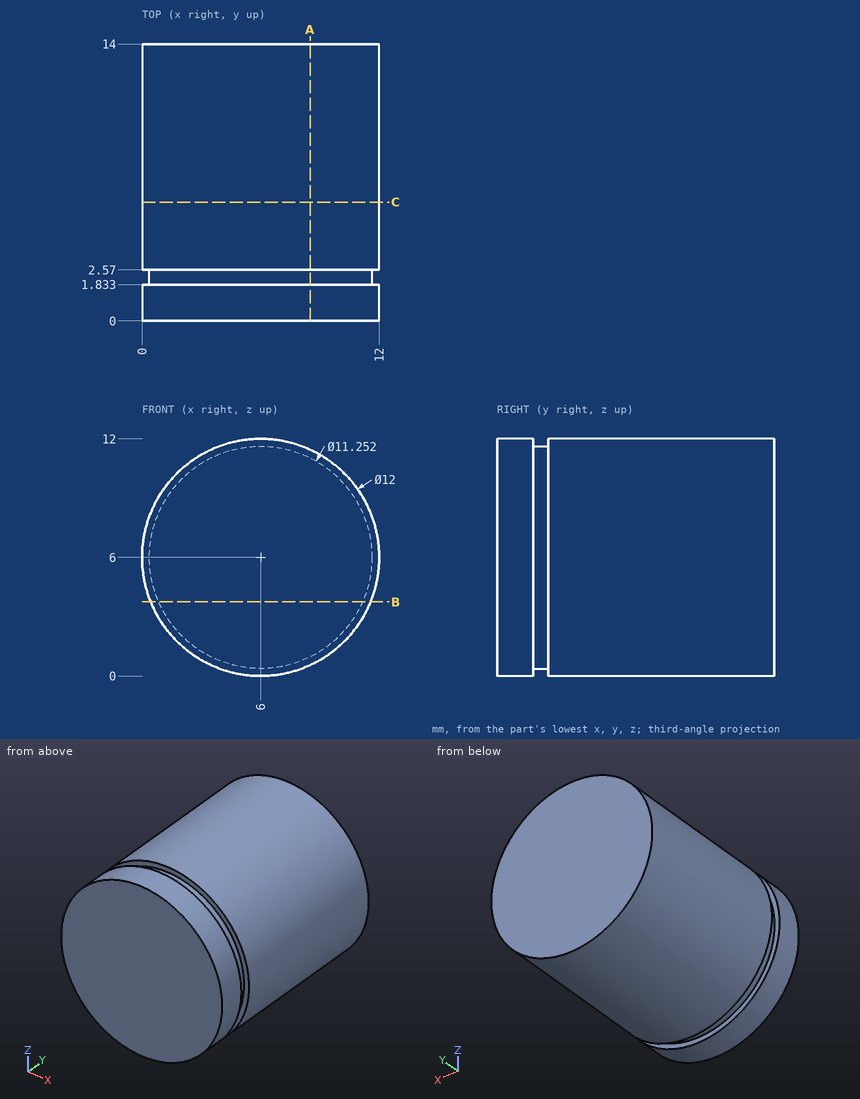
Answer from the drawing. Dimensions are ordinates in mm from the lowest x, y and z of the part. Round coordinates to 2 decimals unless told otherwise and drop trailing zeros. Loops run counter-clockwise (first coordinate to the right, second up) from the corner with the lowest first, then second, coordinate; pieces in that order, holes last.
Q1. Each of these flat-tipped pins is pushed along its axis until it touches: pin 1 (6 mm diameter, centred on y = 8, z = 2.5, fed in from +X); pin 2 (4 mm diameter, centred on y = 11, z = 3, fed in from -X); pin 3 (2 mm diameter, centred on y = 4, z = 10, fed in from +X). Where does it stop, or does it pass through?
Q2. Section C-C on y = 6 is taken. Write down the section's boundary in (x, z).
Q3. Section B-B on z = 3.75 is taken. Write down the section's boundary in (x, y).
Q4. Section A-A on x = 8.5 is taken. Write down the section's boundary in (y, z) (1 decimal).
Q5. Consider probe 1 along Z at (x, y) = (9.75, 2) (1 decimal); probe 2 along X at (y, z) = (11.5, 1) (1 decimal); probe 3 along X at (y, z) = (8, 2.25) (1 decimal). Determine where each line is inside the solid, lowest interval first.
Output:
1. pin 1: stops at x = 11.98
1. pin 2: stops at x = 0.08
1. pin 3: stops at x = 11.2
2. outline: circle Ø12 at (6, 6)
3. outline: (0.44, 0) - (11.56, 0) - (11.56, 1.83) - (11.16, 1.83) - (11.16, 2.57) - (11.56, 2.57) - (11.56, 14) - (0.44, 14) - (0.44, 2.57) - (0.84, 2.57) - (0.84, 1.83) - (0.44, 1.83) - close
4. outline: (0, 0.5) - (1.8, 0.5) - (1.8, 1) - (2.6, 1) - (2.6, 0.5) - (14, 0.5) - (14, 11.5) - (2.6, 11.5) - (2.6, 11) - (1.8, 11) - (1.8, 11.5) - (0, 11.5) - close
5. probe 1: z = 1.8 to 10.2
5. probe 2: x = 2.7 to 9.3
5. probe 3: x = 1.3 to 10.7
